from build123d import *

# Parameters (mm, degrees)
F0_R     = 9.525
F1_DEPTH = 3.175
F2_R     = 6.0325
F3_DEPTH = 9.398
F4_W     = 4.826
F4_H     = 4.826
F5_DEPTH = 11.938


with BuildPart() as f1:
    # F0 (on Top) → F1 (new body)
    with BuildSketch(Plane.XY):
        Circle(F0_R)
    extrude(amount=F1_DEPTH)

    # F2 (on face) → F3 (join)
    with BuildSketch(Plane.XY.offset(3.175)):
        Circle(F2_R)
    extrude(amount=F3_DEPTH)

    # F4 (on face) → F5 (cut)
    with BuildSketch(Plane(origin=(0, 0, 0), x_dir=(1, 0, 0), z_dir=(0, 0, -1))):
        with Locations((0.071996, 0)):
            Rectangle(F4_W, F4_H)
    extrude(amount=-F5_DEPTH, mode=Mode.SUBTRACT)


solid = f1.part
Could you check a few things on this model? Use its own coordinates, in mm. A direction names the side the tool comes from. Give positions to 0.01 mm unless a question says otherwise; leave off trailing zeros. Order: outer loops, then holes, each group sorted by start corner. A loop starts at its lowest first (then second) coordinate and runs counter-clockwise, first axis right, second up.
1. Suppose I cut it at C-C (x = 0). List the corners of the cut face in (y, z) for me (1 decimal), plus the area to 3 significant figures.
2. Will these pins go through, and if not, where does the flat tip stop? P1, Ø3, axis at y = -2.5, z = 4, coming from the -X side; P2, Ø1.4, axis at y = 0, z = 5.5, coming from the -X side; P3, Ø4, axis at y = -1, z = 8.5, coming from the +X side.
3. Suppose I cut it at A-A (z = 1.25). List the corners of the cut face in (x, y) for me (3 decimals), plus the area to 3 significant figures.
4. I need wall thicknesses on L1, parallel to Z at x = 4.25, y = 5 (3 decimals); L2, parallel to X at y = -1.75, z = 9.5 (3 decimals); L3, parallel to X at y = 0.25, z = 8.75 (3 decimals). Which ranges of each line are inside material? Lowest first, please.
5. For faces 1 (the flat face through (-0.1, -6.2, 3.175)), 2 (the flat face through (0, 0, 11.938)), 3 (the flat face through (4, 0, 0)), which set-ups out of +Z, -Z, +X, -X, +Y, -Y let a thin tool reach every point of the face, with its end or its side?
6. We'd pull the mould along X, two halves only. Please class faces 4 (the flat face through (2.485, 0, 6)), 5 (the flat face through (0, 0, 12.573)), 6 (the cylindrical face through (-7.559, -5.796, 1.565)): pulls with the +X half, pulls with the -X half, needs draft (parallel to the pull), parting line crosses it, or undercut.
7. Suppose I cut it at D-D (z = 4.5). List the corners of the cut face in (x, y) for me (1 decimal).
8. Suppose I cut it at B-B (y = 0). List the corners of the cut face in (x, z) for me (1 decimal), plus the area to 3 significant figures.
Solved:
1. outline: (-9.5, 0) - (-2.4, 0) - (-2.4, 11.9) - (2.4, 11.9) - (2.4, 0) - (9.5, 0) - (9.5, 3.2) - (6, 3.2) - (6, 12.6) - (-6, 12.6) - (-6, 3.2) - (-9.5, 3.2) - close
1. area: 116 mm2
2. P1: stops at x = -9.44
2. P2: stops at x = -6.03
2. P3: stops at x = 6.03
3. outline: circle Ø19.05 at (0, 0); hole (-2.341, -2.413) - (2.485, -2.413) - (2.485, 2.413) - (-2.341, 2.413) - close
3. area: 262 mm2
4. L1: z = 0 to 3.175
4. L2: x = -5.773 to -2.341, 2.485 to 5.773
4. L3: x = -6.027 to -2.341, 2.485 to 6.027
5. face 1: +Z
5. face 2: -Z
5. face 3: -Z, +X, -X, +Y, -Y
6. face 4: undercut
6. face 5: needs draft
6. face 6: parting line crosses it
7. outline: circle Ø12.1 at (0, 0); hole (-2.3, -2.4) - (2.5, -2.4) - (2.5, 2.4) - (-2.3, 2.4) - close
8. outline: (-9.5, 0) - (-2.3, 0) - (-2.3, 11.9) - (2.5, 11.9) - (2.5, 0) - (9.5, 0) - (9.5, 3.2) - (6, 3.2) - (6, 12.6) - (-6, 12.6) - (-6, 3.2) - (-9.5, 3.2) - close
8. area: 116 mm2
